from build123d import *

# Parameters (mm, degrees)
F1_DEPTH    = 1.5
F2_DEPTH    = 5.5
F3_DEPTH    = 7
F4_T1_DEPTH = 21.6191756982
F4_T3_DEPTH = 21.6239840214
F5_R        = 1
F6_D        = 3.2
F6_DEPTH    = 4
F6_TIP      = 0.9613769904
F7_D        = 8
F7_DEPTH    = 4
F7_TIP      = 2.4034424761


# Not quite as in the source:
# - a fillet or chamfer that OpenCascade refuses, or shapes differently, is made with other operations: its cross-section is extruded or revolved along the edge and cut away or added


with BuildPart() as f1:
    # F0 (on Top) → F1 (new body)
    with BuildSketch(Plane.XY):
        with BuildLine():
            Line((-66.0687833834, 84.994474126), (-65.6429035596, 87.1528592574))
            ThreePointArc((-65.6429035596, 87.1528592574), (-84.7546054832, 85.2563072371), (-86.3354477268, 66.1159050004))
            Line((-86.3354477268, 66.1159050004), (-84.1804171789, 66.558446905))
            Line((-84.1804171789, 66.558446905), (-79.945453805, 62.3081427722))
            ThreePointArc((-79.945453805, 62.3081427722), (-64.2506598446, 65.1001279098), (-61.7378264361, 80.8420276277))
            Line((-61.7378264361, 80.8420276277), (-66.0687833834, 84.994474126))
        make_face()
    extrude(amount=F1_DEPTH)

    # F0 (on Top) → F2 (join)
    with BuildSketch(Plane.XY):
        Polygon((-84.1804171789, 66.558446905), (-86.3354477268, 66.1159050004), (-86.9652344199, 64.4552756389), (-84.6716307932, 64.9262739357), (-81.0080298382, 61.2494019287), (-79.945453805, 62.3081427722), align=None)
        Polygon((-63.9854566278, 87.8042374119), (-65.6429035596, 87.1528592574), (-66.0687833834, 84.994474126), (-61.7378264361, 80.8420276277), (-60.6997148116, 81.9247668645), (-64.4382903395, 85.5092483194), align=None)
    extrude(amount=F2_DEPTH)

    # F0 (on Top) → F3 (join)
    with BuildSketch(Plane.XY):
        with BuildLine():
            ThreePointArc((-86.3354477268, 66.1159050004), (-84.7546054832, 85.2563072371), (-65.6429035596, 87.1528592574))
            Line((-65.6429035596, 87.1528592574), (-63.9854566278, 87.8042374119))
            ThreePointArc((-63.9854566278, 87.8042374119), (-85.82068996, 86.3115247186), (-86.9652344199, 64.4552756389))
            Line((-86.9652344199, 64.4552756389), (-86.3354477268, 66.1159050004))
        make_face()
    extrude(amount=F3_DEPTH)

    # F4: fillet of radius 6 on 2 edges, made by hand

    # F4_s2 → F4_t1 (cut)
    with BuildSketch(Plane(origin=(6.9172981305, 18.2396174816, 0), x_dir=(0, 0, 1), z_dir=(0.3546014652, 0.9350175404, 0))):
        with BuildLine():
            ThreePointArc((5.5, -104.169954771), (6.6124860802, -106.0172613941), (7, -108.1385817376))
            Line((7, -108.1385817376), (7, -104.169954771))
            Line((7, -104.169954771), (5.5, -104.169954771))
        make_face()
    extrude(amount=F4_T1_DEPTH, mode=Mode.SUBTRACT)

    # F4_s4 → F4_t3 (cut)
    with BuildSketch(Plane(origin=(-36.4260217608, -14.315459745, 0), x_dir=(0, 0, 1), z_dir=(0.9307059478, 0.3657682856, 0))):
        with BuildLine():
            ThreePointArc((5.5, -105.123776774), (6.6124860802, -106.971083397), (7, -109.0924037406))
            Line((7, -109.0924037406), (7, -105.123776774))
            Line((7, -105.123776774), (5.5, -105.123776774))
        make_face()
    extrude(amount=F4_T3_DEPTH, mode=Mode.SUBTRACT)

    # F5 (call 1 of 10: OpenCascade refuses the feature's edges together)
    f5_edges = [f1.edges().sort_by_distance(p)[0] for p in [
        (-86.965234, 64.455276, 2.75),
    ]]
    fillet(f5_edges, radius=F5_R)

    # F5#2 (call 2 of 10)
    f5_2_edges = [f1.edges().sort_by_distance(p)[0] for p in [
        (-84.671631, 64.926274, 2.75),
    ]]
    fillet(f5_2_edges, radius=F5_R)

    # F5#3 (call 3 of 10)
    f5_3_edges = [f1.edges().sort_by_distance(p)[0] for p in [
        (-81.00803, 61.249402, 2.75),
    ]]
    fillet(f5_3_edges, radius=F5_R)

    # F5#4 (call 4 of 10)
    f5_4_edges = [f1.edges().sort_by_distance(p)[0] for p in [
        (-60.699715, 81.924767, 2.75),
    ]]
    fillet(f5_4_edges, radius=F5_R)

    # F5#5 (call 5 of 10)
    f5_5_edges = [f1.edges().sort_by_distance(p)[0] for p in [
        (-64.43829, 85.509248, 2.75),
    ]]
    fillet(f5_5_edges, radius=F5_R)

    # F5#6 (call 6 of 10)
    f5_6_edges = [f1.edges().sort_by_distance(p)[0] for p in [
        (-63.985457, 87.804237, 2.75),
    ]]
    fillet(f5_6_edges, radius=F5_R)

    # F5#7 (call 7 of 10)
    f5_7_edges = [f1.edges().sort_by_distance(p)[0] for p in [
        (-84.180417, 66.558447, 3.5),
    ]]
    fillet(f5_7_edges, radius=F5_R)

    # F5#8 (call 8 of 10)
    f5_8_edges = [f1.edges().sort_by_distance(p)[0] for p in [
        (-66.068783, 84.994474, 3.5),
    ]]
    fillet(f5_8_edges, radius=F5_R)

    # F5#9 (call 9 of 10)
    f5_9_edges = [f1.edges().sort_by_distance(p)[0] for p in [
        (-65.642904, 87.152859, 3.5),
    ]]
    fillet(f5_9_edges, radius=F5_R)

    # F5#10 (call 10 of 10)
    f5_10_edges = [f1.edges().sort_by_distance(p)[0] for p in [
        (-86.335448, 66.115905, 3.5),
    ]]
    fillet(f5_10_edges, radius=F5_R)

    # F6
    with Locations(Plane(origin=(0, 0, 0), x_dir=(1, 0, 0), z_dir=(0, 0, -1))):
        with Locations((-83.5608274937, -74.7376042604), (-74.0608274937, -82.7376042604), (-64.5608274937, -74.7376042604), (-74.0608274937, -66.7376042604)):
            Hole(F6_D / 2, depth=F6_DEPTH)
            with Locations((0, 0, -(F6_DEPTH + F6_TIP / 2))):  # 118° drill point
                Cone(0, F6_D / 2, F6_TIP, mode=Mode.SUBTRACT)

    # F7
    with Locations(Plane(origin=(0, 0, 0), x_dir=(1, 0, 0), z_dir=(0, 0, -1))):
        with Locations((-74.0608274937, -74.7376042604)):
            Hole(F7_D / 2, depth=F7_DEPTH)
            with Locations((0, 0, -(F7_DEPTH + F7_TIP / 2))):  # 118° drill point
                Cone(0, F7_D / 2, F7_TIP, mode=Mode.SUBTRACT)


solid = f1.part
Input: part model. Units: mm. Frame: model coordinates. A direction names the side the tool comes from. Round coordinates to 2 decimals unless told otherwise and drop trailing zeros. Loops run counter-clockwise (first coordinate to the right, second up) from the corner with the lowest first, then second, coordinate; pieces in that order, holes last. Notation, with made-up numbers: M 5,14.25 L 22,14.25 A19 cw 22,46.25 Z; hole C 78,42 d11. An arc over 180 degrees is marked long. Answer as CSV lines item,"result". Start each with the question number.
(1) Section A-A, the plane x = -73.5. Output: boundary loops of the cut face in (y, z).
(2) Line query: line 1 (Y direction, x = -86.5, z = 3.5); line 2 (X direction, y = 88, z = 2.5); line 3 (Z direction, x = -68, y = 79.5). Output: solid intervals per line, ascending. Write a range as [from, to].
(3) First-contact query: pin 1 (2.5 mm diameter, centred on x = -64, y = 85, fed in from +Z); pin 2 (8.5 mm diameter, centred on x = -74.5, y = 75, fed in from +Z); pin 3 (1 mm diameter, centred on x = -79.5, y = 67.5, fed in from -Z); pin 4 (1.5 mm diameter, centred on x = -71, z = 4, fed in from -Y). Flat tips, straight axial feed; report the tip coordinate or a pass-through.
(4) Reachability of faces 1 (the cylindrical face through (-85, 85, 4)), 2 (the flat face through (-81.85, 64.22, 3.47)), 3 (the flat face through (-63.733, 82.755, 3.472)) from +Z, -Z, +X, -X, +Y, -Y: full face, straight path, thin tool, end or side. Return the list, or none.
(5) Section C-C, the plane y = 77. Output: boundary loops of the cut face in (x, z).
(6) Draft query along X for faces 4 (the cylindrical face through (-61.114, 81.905, 2.788)), 5 (the cylindrical face through (-84.213, 66.426, 3.528)), 6 (the cylindrical face through (-85.59, 86.54, 3.45)). Return one class per face: released by +X, released by -X, zero draft, split by the parting line, or undercut.
(7) Section B-B, the plane z = 4. Output: boundary loops of the cut face in (x, y), plus the area to 3 significant figures.
(8) Section D-D, the plane x = -77. Output: boundary loops of the cut face in (y, z).
Values found:
1,outline,"M 61,0 L 65.24,0 L 65.24,1.5 L 61,1.5 Z; M 68.24,0 L 70.78,0 L 70.78,1.5 L 68.24,1.5 Z; M 78.7,0 L 81.24,0 L 81.24,1.5 L 78.7,1.5 Z; M 84.24,0 L 91.23,0 L 91.23,7 L 89.73,7 L 89.73,1.5 L 84.24,1.5 Z"
2,line 1,"y = [64.56, 66.45], [83.12, 85.58]"
2,line 2,"x = [-83.88, -81.07], [-67.05, -64.31]"
2,line 3,"z = [0, 1.5]"
3,pin 1,"stops at z = 5.5"
3,pin 2,"stops at z = 1.5"
3,pin 3,"stops at z = 0"
3,pin 4,"stops at y = 89.25"
4,face 1,"+Z"
4,face 2,"+Z, +X"
4,face 3,"+Z, -Y"
5,outline,"M -90.4,0 L -77.36,0 L -77.36,1.5 L -88.89,1.5 L -88.89,7 L -90.4,7 Z; M -70.76,0 L -60.5,0 L -60.5,1.5 L -70.76,1.5 Z"
6,face 4,"released by +X"
6,face 5,"undercut"
6,face 6,"split by the parting line"
7,outline,"M -87.36,64.97 A1 ccw -86.35,64.58 L -85.2,64.82 A1 cw -84.29,64.54 L -81.71,61.96 A1 ccw -80.3,61.96 L -79.95,62.31 L -83.8,66.18 A1 ccw -84.71,66.45 L -85.68,66.25 A1 cw -86.72,66.69 A15 cw -66.23,87.53 A1 cw -65.77,86.49 L -65.96,85.53 A1 ccw -65.67,84.62 L -61.74,80.84 L -61.39,81.2 A1 ccw -61.42,82.62 L -64.04,85.13 A1 cw -64.33,86.05 L -64.11,87.18 A1 ccw -64.51,88.19 A16.5 ccw Z"
7,area,"90.4 mm²"
8,outline,"M 61.3,0 L 72.02,0 L 72.02,1.5 L 61.3,1.5 Z; M 77.45,0 L 90.97,0 L 90.97,7 L 89.45,7 L 89.45,1.5 L 77.45,1.5 Z"
